Study the drawing (mm; zero at the part's minimum x, y, z) and answer. Round coordinates to 2 decimals unless told otherwise and drop trailing zeros. Loops run counter-clockwise (first coordinate to the right, second up) from the corner with the lowest first, then second, coordinate; pieces in that order, holes last. Notation, with made-up numbers: (30, -27.75) - (81, -27.75) arc R17 ccw to (81, -6.75) - close; hole circle Ø11 at (47.5, -27). An arc over 180 degrees is marked (long way). Use CSV: the item, a comma, the result in double quotes. Start each with the question number.
1. Consider line 1 along X through (y, z) = (3.6, 7.75); line 2 along X through (y, z) = (0.45, 6); line 3 along Z through (x, y) = (2.5, 3.35). Determine where each line is inside the solid, lowest interval first.
2. Determine the mould class of the marked faces 1, 2 and 3 for opening direction X: +X half, -X half, draft (parallel to the pull), parting line (faces both ways), or undercut.
3. Find section C-C (y = 2.3). Give the vertices of the cut face in (x, z).
4. Given pin 1 Ø1.5 at (y, z) = (1, 3.5) entering from -X; pin 2 Ø1 at (x, y) = (6.5, 3.5) entering from +Z, each flat-ended and moving along its own axis, determine where each tip first touches the part or whether it passes through.
5. Find section A-A (x = 5). State how many separate pieces and enclosed holes the cut face has, and give its area (3 significant figures).
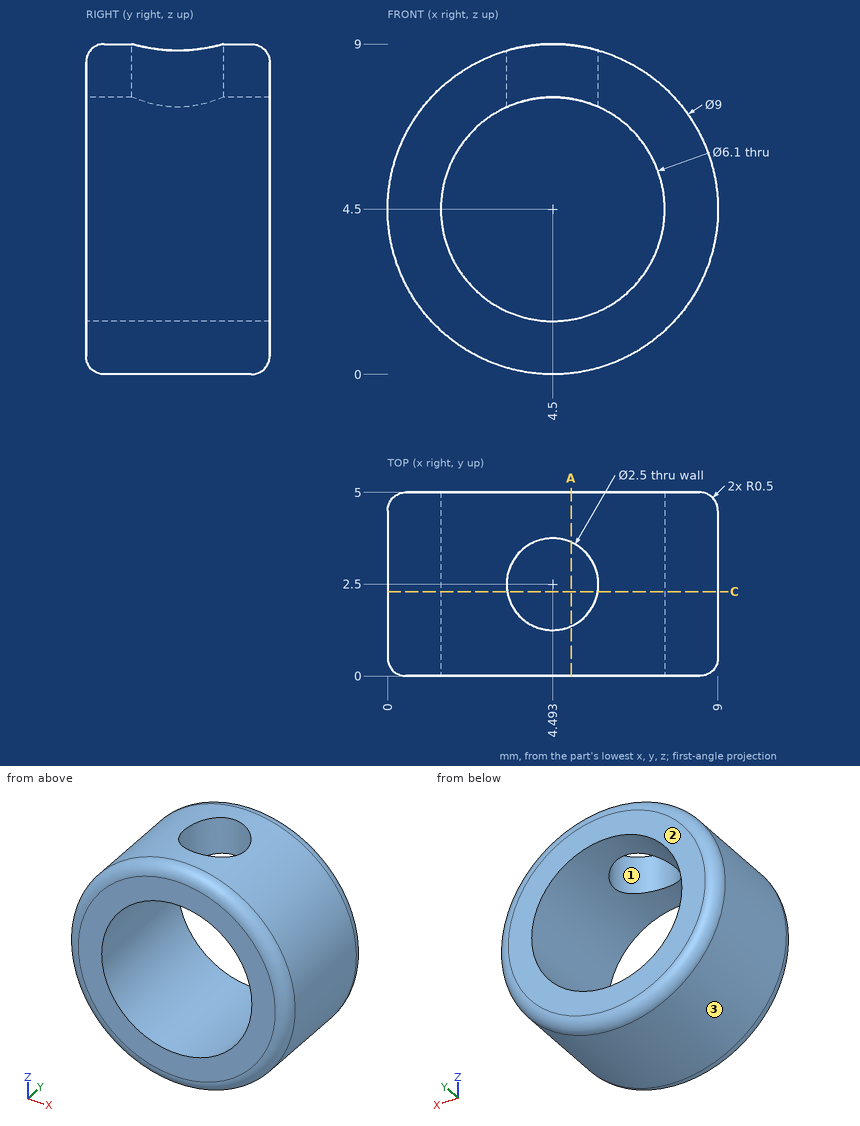
Filled sheet:
1,line 1,"x = 1.39 to 3.9, 5.09 to 7.61"
1,line 2,"x = 0.26 to 1.84, 7.16 to 8.74"
1,line 3,"z = 0.47 to 2.2, 6.8 to 8.53"
2,face 1,"undercut"
2,face 2,"draft"
2,face 3,"parting line"
3,outline,"(3.26, 7.29) - (3.26, 8.83) arc R4.5 ccw (long way) to (5.73, 8.83) - (5.73, 7.29) arc R3.05 cw (long way) to start"
4,pin 1,"stops at x = 0.01"
4,pin 2,"stops at z = 8.74"
5,separate pieces,"3"
5,enclosed holes,"0"
5,area,"11.1 mm²"
